from build123d import *

# Parameters (mm, degrees)
SKETCH1_W           = 30
SKETCH1_H           = 30
BOSS_EXTRUDE1_DEPTH = 500
SKETCH2_R           = 15
BOSS_EXTRUDE2_DEPTH = 30
SKETCH4_R           = 10
CUT_EXTRUDE1_DEPTH  = 50


with BuildPart() as part:
    # Sketch1 → Boss-Extrude1 (new body)
    with BuildSketch(Plane(origin=(0, 0, 0), x_dir=(1, 0, 0), z_dir=(0, 1, 0))):
        Rectangle(SKETCH1_W, SKETCH1_H)
    extrude(amount=BOSS_EXTRUDE1_DEPTH)

    # Sketch2 → Boss-Extrude2 (add)
    with BuildSketch(Plane.XY.offset(15)):
        with Locations((0, 500)):
            Circle(SKETCH2_R)
    extrude(amount=-BOSS_EXTRUDE2_DEPTH)

    # Sketch4 → Cut-Extrude1 (cut)
    with BuildSketch(Plane.XZ):
        Circle(SKETCH4_R)
    extrude(amount=-CUT_EXTRUDE1_DEPTH, mode=Mode.SUBTRACT)


solid = part.part
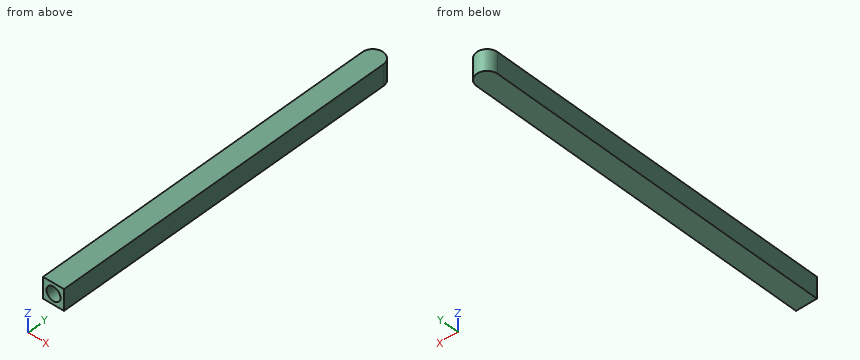
Build history of the part. All positions in model axes, mm. Round coordinates to 2 decimals unless told otherwise and drop trailing zeros. Write each loop counter-clockwise with the first axis right and the second up, starting at its lowest first coordinate (ties: lowest second). Pieces come first, ordered by that corner, then holes. Notation, with made-up numbers: M -19,-8.75 L 32,-8.75 A18 cw 32,23.25 Z; hole C -23.5,73 d5. An arc over 180 degrees is marked long. Answer as a JSON object with one key per item and string values. Group by question number.
(1) Flat gauge pins, fed straight in: pin 1 (2 mm diameter, centred on x = 6, z = 4.5, fed in from -Y); pin 2 (8 mm diameter, centred on x = 7, z = -9.5, fed in from +Y). Where does each tip first touch, or does it go through?
(2) Cut at B-B (z = 0). Give the cut face in (x, y), and give its area (3 significant figures).
(3) Drill centre lines: L1, parallel to Z at x = 0, y = 20; L2, parallel to Y at x = 3.5, z = 9.5; L3, parallel to Y at x = 4, z = -3. Where is each one in solid material? Low to high.
(4) Cut at A-A (x = 0). Give the cut face in (y, z).
Responses:
{
 "1": {"pin 1": "stops at y = 50", "pin 2": "stops at y = 514.7"},
 "2": {"outline": "M -15,0 L -10,0 L -10,50 L 10,50 L 10,0 L 15,0 L 15,500 A15 ccw -15,500 Z", "area": "14,400 mm2"},
 "3": {"L1": "z = -15 to -10, 10 to 15", "L2": "y = 0 to 514.59", "L3": "y = 50 to 514.46"},
 "4": {"outline": "M 0,-15 L 515,-15 L 515,15 L 0,15 L 0,10 L 50,10 L 50,-10 L 0,-10 Z"}
}
